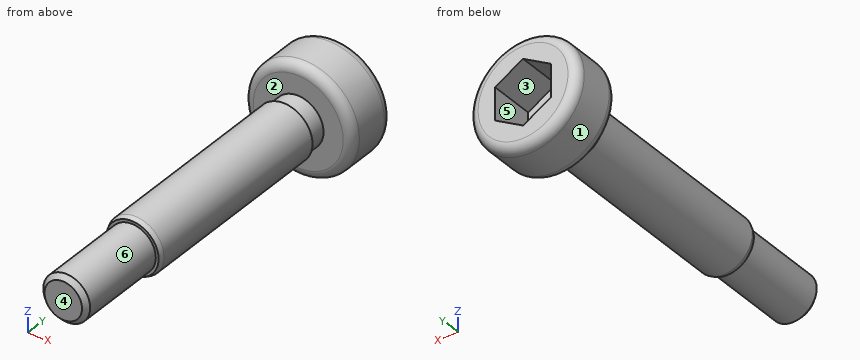
from build123d import *

# Parameters (mm, degrees)
SKETCH_2_R          = 1.25
EXTRUDE_1_DEPTH     = 4.75
SKETCH_3_R          = 1.25
EXTRUDE_2_DEPTH     = 0.25
EXTRUDE_2_TAPER     = 45
CUT_EXTRUDE_1_DEPTH = 2.4
FILLET_1_R          = 0.5


with BuildPart() as part:
    # 草图1 → 旋转1 (revolve)
    with BuildSketch(Plane(origin=(0, 0, 0), x_dir=(-1, 0, 0), z_dir=(0, 0, -1))):
        Polygon((-1.4, -14.8), (0, -14.8), (0, 0), (-2.9, 0), (-2.9, -2.8), (-1.35, -2.8), (-1.35, -3.8), (-1.5, -3.8), (-1.5, -14.55), align=None)
    revolve(axis=Axis((0, -14.8, 0), (0, 1, 0)))

    # 草图2 → 凸台-拉伸1 (add)
    with BuildSketch(Plane.XZ.offset(14.8)):
        Circle(SKETCH_2_R)
    extrude(amount=EXTRUDE_1_DEPTH)

    # 草图3 → 凸台-拉伸2 (add)
    with BuildSketch(Plane.XZ.offset(19.55)):
        Circle(SKETCH_3_R)
    extrude(amount=EXTRUDE_2_DEPTH, taper=EXTRUDE_2_TAPER)

    # 草图4 → 切除-拉伸1 (cut)
    with BuildSketch(Plane(origin=(0, 0, 0), x_dir=(-1, 0, 0), z_dir=(0, 1, 0))):
        Polygon((-1.5, 0.866025404), (-1.5, -0.866025404), (0, -1.732050808), (1.5, -0.866025404), (1.5, 0.866025404), (0, 1.732050808), align=None)
    extrude(amount=-CUT_EXTRUDE_1_DEPTH, mode=Mode.SUBTRACT)

    # 圆角1
    fillet_1_edges = [part.edges().sort_by_distance(p)[0] for p in [
        (-2.9, -2.8, 0),
        (-2.9, 0, 0),
    ]]
    fillet(fillet_1_edges, radius=FILLET_1_R)


solid = part.part
Design review of the part built by this model. Coordinates are the model's own, in mm. Face numbers are marked on the shaded views. A direction names the side the tool comes from. Give positions to 0.01 mm unless a question says otherwise; leave off trailing zeros. Loops run counter-clockwise (first coordinate to the right, second up) from the corner with the lowest first, then second, coordinate; pieces in that order, holes last. Notation, with made-up numbers: (-35, 61.5) -> (-22, 61.5) arc R19 cw to (-22, 65.5) -> close; hole circle Ø9 at (62, -16). An arc over 180 degrees is marked (long way). One line per question, with ' | ' between items. Start each with the question number.
(1) For line 1 (Y direction, x = 0.45, z = 2.35); line 2 (X direction, y = -10, z = 0.55); line 3 (Y direction, x = 0.35, z = 0.8), list the stretches that pass through material, from the lowest coordinate up.
(2) Insertion check: P1, Ø0.9, axis at x = -0.5, z = -0.5, coming from the +Y side; P2, Ø2, axis at x = -2, z = 2, coming from the -Y side; P3, Ø3, axis at y = -15, z = 0.5, coming from the -X side. Each pin has a flat end and moves straight along its axis. Give the tip position at first contact, or say it passes through.
(3) For the marked faces 4, 5 and 6, list the 3-axis set-ups (+Z, -Z, +X, -X, +Y, -Y) from which the entire face can be reached by the end or side of a thin tool; tool diameter is ignored.
(4) Draft analysis for pull direction X (two halves, no side actions). For the marked faces 1, 2 and 3, state which applies: +X half, -X half, draft (parallel to the pull), parting line (faces both ways), or undercut.
(5) We need section B-B (y = -6.5). State the section outline as (x, z) points, and give its area (3 significant figures).
(6) We need section A-A (y = -15.75). State the section outline as (x, z) points, and give its area (3 significant figures).
The answers:
1) line 1: y = -2.8 to 0 | line 2: x = -1.4 to 1.4 | line 3: y = -19.8 to -2.4
2) P1: stops at y = -2.4 | P2: stops at y = -2.8 | P3: stops at x = -1.5
3) face 4: +Z, -Z, +X, -X, -Y | face 5: +Y | face 6: -Y
4) face 1: parting line | face 2: draft | face 3: undercut
5) outline: circle Ø3 at (0, 0) | area: 7.07 mm^2
6) outline: circle Ø2.5 at (0, 0) | area: 4.91 mm^2
